Check sheet for the modelled part. Datum: model origin and axes. Units: mm. Give positions to 0.01 mm unless a question says otherwise; leave off trailing zeros. Order: outer loops, then holes, each group sorted by start corner. A loop starts at its lowest first (then second) coordinate and runs counter-clockwise, first axis right, second up. Notation, with made-up numbers: (25.25, 44.5) -> (83.25, 44.5) arc R25 cw to (83.25, 64.5) -> close; hole circle Ø6 at (-29, 30). An arc over 180 degrees is marked (long way). One line per question, with ' | ' between items. Start each with the question number.
Autodesk Inventor part; units mm, degrees
ref_plane "YZ Plane" through (0, 0, 0) normal (1, 0, 0) x (0, 1, 0)
ref_plane "XZ Plane" through (0, 0, 0) normal (0, 1, 0) x (-1, 0, 0)
ref_plane "XY Plane" through (0, 0, 0) normal (0, 0, 1) x (1, 0, 0)
sketch "main" plane through (0, 0, 0) normal (0, 0, 1) x (1, 0, 0)
  circle A0 centre (15.4343, 10.6591) radius 2.1844
  circle A1 centre (6.35, -22.225) radius 2.15
  circle A2 centre (-9.9657, 10.6591) radius 2.1844
  circle A3 centre (15.4343, -6.35) radius 2.0955
  arc A4 (19.5678, -8.7154) -> (20.176, -6.7945) centre (15.4343, -6.35) ccw
  arc A5 (21.7565, 10.0664) -> (15.4343, 17.0091) centre (15.4343, 10.6591) ccw
  arc A6 (-9.9657, 17.0091) -> (-15.5267, 7.5934) centre (-9.9657, 10.6591) ccw
  arc A7 (2.1793, -24.5243) -> (10.4836, -24.5904) centre (6.35, -22.225) ccw
  line L0 (21.7565, 10.0664) -> (20.176, -6.7945)
  line L1 (15.4343, 17.0091) -> (-9.9657, 17.0091)
  line L2 (-15.5267, 7.5934) -> (2.1793, -24.5243)
  line L3 (19.5678, -8.7154) -> (10.4836, -24.5904)
  line L4 (7.8311, -10.0478) -> (10.6181, -5.1775)
  line L5 (10.8208, -4.5372) -> (11.785, 5.7484)
  line L6 (10.2044, 7.4841) -> (-1.902, 7.4841)
  line L7 (-3.2922, 5.1301) -> (5.063, -10.0258)
  arc A8 (10.6181, -5.1775) -> (10.8208, -4.5372) centre (9.2402, -4.389) ccw
  arc A9 (5.063, -10.0258) -> (7.8311, -10.0478) centre (6.4532, -9.2594) ccw
  arc A10 (-1.902, 7.4841) -> (-3.2922, 5.1301) centre (-1.902, 5.8966) ccw
  arc A11 (11.785, 5.7484) -> (10.2044, 7.4841) centre (10.2044, 5.8966) ccw
  circle A12 centre (-2.909, -6.39) radius 2.0955
  point P0 (7.047, 1.8005)
  dimension "d0" = 4.191
  dimension "d1" = 12.7
  dimension "d2" = 12.7
  dimension "d3" = 9.525
  dimension "d4" = 9.525
  dimension "d5" = 1.5875
  dimension "d8" = 4.7625
  dimension "d9" = 4.191
sketch "Sketch1" plane through (0, 0, 0) normal (0, 1, 0) x (-1, 0, 0)
  circle A0 centre (0, 0) radius 2.1844
  circle A1 centre (32.891, -9.0591) radius 2.15
  circle A2 centre (0.0195, -25.4) radius 2.1844
  circle A3 centre (17.0091, 0.013) radius 2.0955
  arc A4 (19.3713, 4.1484) -> (17.4499, 4.7551) centre (17.0091, 0.013) ccw
  arc A5 (0.5878, 6.3227) -> (-6.35, -0.0049) centre (0, 0) ccw
  arc A6 (-6.3305, -25.4049) -> (3.0894, -30.9586) centre (0.0195, -25.4) ccw
  arc A7 (35.1935, -13.228) -> (35.2532, -4.9237) centre (32.891, -9.0591) ccw
  line L0 (0.5878, 6.3227) -> (17.4499, 4.7551)
  line L1 (-6.35, -0.0049) -> (-6.3305, -25.4049)
  line L2 (3.0894, -30.9586) -> (35.1935, -13.228)
  line L3 (19.3713, 4.1484) -> (35.2532, -4.9237)
  line L4 (20.7127, -7.5873) -> (15.8402, -4.804)
  line L5 (15.1998, -4.6018) -> (4.9135, -3.6455)
  line L6 (3.179, -5.2274) -> (3.1883, -17.3338)
  line L7 (5.5433, -18.7222) -> (20.6928, -10.3554)
  arc A8 (15.8402, -4.804) -> (15.1998, -4.6018) centre (15.0528, -6.1825) ccw
  arc A9 (20.6928, -10.3554) -> (20.7127, -7.5873) centre (19.9253, -8.9657) ccw
  arc A10 (3.1883, -17.3338) -> (5.5433, -18.7222) centre (4.7758, -17.3326) ccw
  arc A11 (4.9135, -3.6455) -> (3.179, -5.2274) centre (4.7665, -5.2262) ccw
  circle A12 centre (17.0631, -18.3302) radius 2.0955
  point P0 (0, 0)
extrude "Extrusion1" add sketch "Sketch1" along normal blind 1.5875
properties part number "mount" material "Acetal Resin, White"
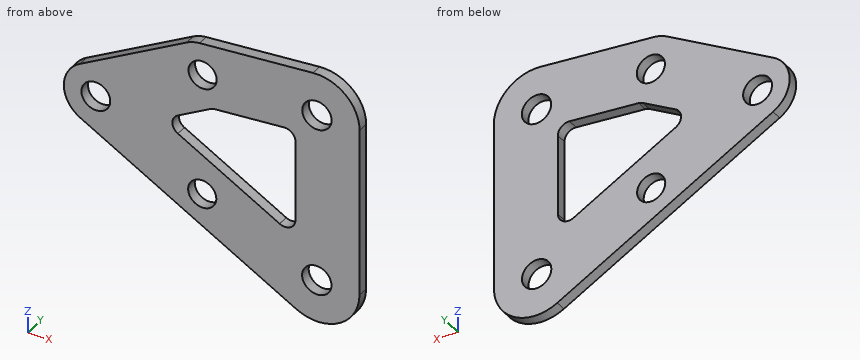
1. Cross-section at C-C on y = 1.1. Record the boundary of the cut face in (x, z), and give its area (3 significant figures).
2. Go/stop test with a flat-tipped pin: pin 1 (8 mm diameter, centred on x = -15.5, z = -15, fed in from -Y). Record where the tip stops, or that it passes through.
3. Cross-section at D-D on x = -7. Record the boundary of the cut face in (y, z), and give its area (3 significant figures).
4. Scan lines: probe 1 along X at (y, z) = (1.4, -9); probe 2 along X at (y, z) = (0.25, -17); probe 3 along Z at (x, y) = (1, 1.55). Record each from-to range of solid material in increasing order.
5. Cross-section at A-A on x = 0. Record the boundary of the cut face in (y, z), and give its area (3 significant figures).
6. Cross-section at B-B on z = -26. Record the boundary of the cut face in (x, y).
Response values:
1) outline: (-35.25, -4.92) arc R4.76 ccw to (-35.19, -13.23) -> (-3.09, -30.96) arc R6.35 ccw to (6.33, -25.4) -> (6.35, 0) arc R6.35 ccw to (-0.59, 6.32) -> (-17.45, 4.76) arc R4.76 ccw to (-19.37, 4.15) -> close; hole circle Ø4.3 at (-32.89, -9.06); hole (-20.71, -7.59) arc R1.59 ccw to (-20.69, -10.36) -> (-5.54, -18.72) arc R1.59 ccw to (-3.19, -17.33) -> (-3.18, -5.23) arc R1.59 ccw to (-4.91, -3.65) -> (-15.2, -4.6) arc R1.59 ccw to (-15.84, -4.8) -> close; hole circle Ø4.19 at (-17.06, -18.33); hole circle Ø4.19 at (-17.01, 0.01); hole circle Ø4.37 at (-0.02, -25.4); hole circle Ø4.37 at (0, 0) | area: 890 mm²
2) pin 1: stops at y = 0
3) outline: (0, -28.8) -> (1.59, -28.8) -> (1.59, -17.92) -> (0, -17.92) -> close; (0, -3.84) -> (1.59, -3.84) -> (1.59, 5.73) -> (0, 5.73) -> close | area: 32.5 mm²
4) probe 1: x = -37.65 to -35.04, -30.74 to -21.51, -3.18 to 6.34 | probe 2: x = -28.36 to -18.68, -15.44 to -8.66, -3.19 to 6.34 | probe 3: z = -31.67 to -27.33, -23.47 to -1.94, 1.94 to 6.27
5) outline: (0, -31.75) -> (1.59, -31.75) -> (1.59, -27.58) -> (0, -27.58) -> close; (0, -23.22) -> (1.59, -23.22) -> (1.59, -2.18) -> (0, -2.18) -> close; (0, 2.18) -> (1.59, 2.18) -> (1.59, 6.35) -> (0, 6.35) -> close | area: 46.6 mm²
6) outline: (-12.07, 0) -> (-2.12, 0) -> (-2.12, 1.59) -> (-12.07, 1.59) -> close; (2.08, 0) -> (6.3, 0) -> (6.3, 1.59) -> (2.08, 1.59) -> close
